The model under review builds one solid part; all positions refer to its coordinate system, in mm. A direction names the side the tool comes from. Give positions to 0.01 mm unless a question says otherwise; leave off trailing zeros. Loops run counter-clockwise (first coordinate to the right, second up) from the corner with the lowest first, then second, coordinate; pieces in that order, holes last. Notation, with made-up numbers: M 41,-6 L 71,-6 A17 cw 71,20 Z; hole C 33.25,63 d1. An arc over 180 degrees is marked long. Put each result on its own line as item: value. Start each with the question number.
```python
from build123d import *

# Parameters (mm, degrees)
F0_W     = 114.3
F0_H     = 114.3
F2_DEPTH = 25.4
F3_W     = 102.25038
F3_H     = 101.6
F4_DEPTH = 19.05
F5_R     = 1.5
F6_DEPTH = 110.49


with BuildPart() as f2:
    # F0 (on Front) → F2 (new body)
    with BuildSketch(Plane.XZ):
        Rectangle(F0_W, F0_H)
    extrude(amount=F2_DEPTH)

    # F3 (on face) → F4 (cut)
    with BuildSketch(Plane.XZ.offset(25.4)):
        with Locations((0.32519, 0)):
            Rectangle(F3_W, F3_H)
    extrude(amount=-F4_DEPTH, mode=Mode.SUBTRACT)

    # F5 (on face) → F6 (cut)
    with BuildSketch(Plane(origin=(0, 0, -57.15), x_dir=(1, 0, 0), z_dir=(0, 0, -1))):
        with Locations((0.175, 16.318)):
            Circle(F5_R)
        with Locations((27.71, 16.318)):
            Circle(F5_R)
        with Locations((-27.71, 16.318)):
            Circle(F5_R)
    extrude(amount=-F6_DEPTH, mode=Mode.SUBTRACT)


solid = f2.part
```
Item 1: Tool access review of faces 5 (the cylindrical face through (-28.9, -15.405, 52.052)), 6 (the flat face through (-51, -25.4, 9)), 7 (the flat face through (-50.8, -16, -1)): name each direction out of +Z, -Z, +X, -X, +Y, -Y from which nothing blocks a thin tool from reaching the whole face with its end or side.
Item 2: Consider section C-C, the plane z = 29. Write out the cut boundary in (x, y), plus the area to 3 significant figures.
Item 3: Draft analysis for pull direction Y (two halves, no side actions). For faces 1 (the flat face through (0, -6.35, 1)), 2 (the flat face through (28, -16, 53.34)), 3 (the flat face through (-1, 0, 1)), 4 (the flat face through (57.15, -13, -1)), state which applies: +Y half, -Y half, draft (parallel to the pull), parting line (faces both ways), or undercut.
Item 4: Consider section A-A, the plane x = 27.71. Write out the cut boundary in (y, z), plus the area to 3 significant figures.
Item 5: To check wall thickness, follow L1, parallel to Z at x = 50, y = -22; L2, parallel to X at y = -16.5, z = -1; L3, parallel to Y at x = 39, z = 48. State the ranges of each line that lie inside material, in increasing order. Write a range as [from, to].
Item 6: Consider section B-B, the plane x = -15.5. Write out the cut boundary in (y, z), plus the area to 3 significant figures.
Item 7: Clearance check with flat-ended pins moving along their axes: pin 1 Ø2.5 at (x, y) = (-27.5, -16) entering from -Z; pin 2 Ø12 at (x, z) = (-13, 42) entering from -Y. State where each tip first meets the part, or that it passes through.
Report:
1. face 5: -Z
1. face 6: +Z, -Z, +X, -X, -Y
1. face 7: -Y
2. outline: M -57.15,-25.4 L -50.8,-25.4 L -50.8,-6.35 L 51.45,-6.35 L 51.45,-25.4 L 57.15,-25.4 L 57.15,0 L -57.15,0 Z
2. area: 955 mm²
3. face 1: -Y half
3. face 2: undercut
3. face 3: +Y half
3. face 4: draft
4. outline: M -25.4,-57.15 L -17.82,-57.15 L -17.82,-50.8 L -25.4,-50.8 Z; M -25.4,50.8 L -17.82,50.8 L -17.82,53.34 L -14.82,53.34 L -14.82,50.8 L -6.35,50.8 L -6.35,-50.8 L -14.82,-50.8 L -14.82,-57.15 L 0,-57.15 L 0,57.15 L -25.4,57.15 Z
4. area: 941 mm²
5. L1: [-57.15, -50.8], [50.8, 57.15]
5. L2: [-57.15, -50.8], [51.45, 57.15]
5. L3: [-6.35, 0]
6. outline: M -25.4,-57.15 L 0,-57.15 L 0,57.15 L -25.4,57.15 L -25.4,50.8 L -6.35,50.8 L -6.35,-50.8 L -25.4,-50.8 Z
6. area: 968 mm²
7. pin 1: z = -57.15
7. pin 2: y = -6.35
